from build123d import *

# Parameters (mm, degrees)
F0_R           = 6.35
F1_DEPTH       = 5
F3_D           = 8
F3_CSINK_D     = 10
F3_CSINK_ANGLE = 90


with BuildPart() as f1:
    # F0 (on Top) → F1 (new body)
    with BuildSketch(Plane.XY):
        with BuildLine():
            Line((-10, 65), (-10, 23.348662))
            ThreePointArc((-10, 23.348662), (-21.997045, 12.7), (-25.220534, -3.014077))
            Line((-25.220534, -3.014077), (-61.291651, -23.839746))
            Line((-61.291651, -23.839746), (-51.291651, -41.160254))
            Line((-51.291651, -41.160254), (-15.220534, -20.334585))
            ThreePointArc((-15.220534, -20.334585), (0, -25.4), (15.220534, -20.334585))
            Line((15.220534, -20.334585), (51.291651, -41.160254))
            Line((51.291651, -41.160254), (61.291651, -23.839746))
            Line((61.291651, -23.839746), (25.220534, -3.014077))
            ThreePointArc((25.220534, -3.014077), (21.997045, 12.7), (10, 23.348662))
            Line((10, 23.348662), (10, 65))
            Line((10, 65), (-10, 65))
        make_face()
        with Locations((-12.990381, -7.5)):
            Circle(F0_R, mode=Mode.SUBTRACT)
        with Locations((12.990381, -7.5)):
            Circle(F0_R, mode=Mode.SUBTRACT)
        with Locations((0, 15)):
            Circle(F0_R, mode=Mode.SUBTRACT)
    extrude(amount=F1_DEPTH)

    # F3 (through all)
    with Locations(Plane.XY.offset(5)):
        with Locations((0, 57), (0, 41), (35.507042, -20.5), (49.363448, -28.5), (-35.507042, -20.5), (-49.363448, -28.5)):
            CounterSinkHole(F3_D / 2, F3_CSINK_D / 2, counter_sink_angle=F3_CSINK_ANGLE)


solid = f1.part
Geometry: final body of the model. Coordinates: model frame, mm. A direction names the side the tool comes from. Give positions to 0.01 mm unless a question says otherwise; leave off trailing zeros. Loops run counter-clockwise (first coordinate to the right, second up) from the corner with the lowest first, then second, coordinate; pieces in that order, holes last. Notation, with made-up numbers: M 79.5,-8 L 127.5,-8 A15 ccw 127.5,19 Z; hole C 36.5,8 d8. An arc over 180 degrees is marked long. Put each result on its own line as item: value. Start each with the question number.
1) Ray query, line 1 along Y through (x, z) = (0, 2.7); line 2 along X through (y, z) = (-7, 2); line 3 along X through (y, z) = (-20.5, 3.1). Return the intervals inside material, ascending.
2) Access query for faces 1 (the flat face through (10, 44, 2)), 2 (the flat face through (-10, 44, 2)), 3 (the flat face through (-33.509, -30.893, 2.465)), 4 (the cylindrical face through (0.867, 53.095, 1.972)). Directions: +Z, -Z, +X, -X, +Y, -Y. A direction counts if a zero-diameter tool reaches every point of the face in a straight line with its end or side. Return the directions, or none.
3) Contact query for flat-ended pins moving along their axis: pin 1 (6.5 mm diameter, centred on x = 49.36, y = -28.5, fed in from -Z); pin 2 (2 mm diameter, centred on x = 47.5, z = 4.5, fed in from +Y); pin 3 (3 mm diameter, centred on x = -33.5, z = 3.5, fed in from +Y); pin 4 (3 mm diameter, centred on x = -45, z = 2.5, fed in from +Y). Output: stop coordinate, or through.
4) Cut plane B-B (y = 41). Output: boundary loops of the cut face in (x, z), then the cut area to 3 significant figures.
5) Cut plane D-D (y = 15). Output: boundary loops of the cut face in (x, z), then the cut area to 3 significant figures.
6) Pull-direction query (Y, two-part tool) for faces 5 (the cylindrical face through (53.36, -28.32, 1.97)), 6 (the flat face through (56.222, -32.621, 2.465)), 7 (the flat face through (0, 4, 0)); classes: pulls with the +Y half, pulls with the -Y half, needs draft (parallel to the pull), parting line crosses it, or undercut.
7) Cut plane C-C (y = -7.5). Output: boundary loops of the cut face in (x, z), then the cut area to 3 significant figures.
8) Cut plane A-A (z = 3.25). Give the number of separate pieces and of enclosed holes in the cut face, then the cut area to 3 significant figures.
Verdict:
1. line 1: -25.4 to 8.65, 21.35 to 37, 45 to 53, 61 to 65
1. line 2: -32.12 to -19.32, -6.66 to 6.66, 19.32 to 32.12
1. line 3: -55.51 to -39.51, -31.51 to -15.51, -15 to 15, 15.51 to 31.51, 39.51 to 55.51
2. face 1: +Z, -Z, +X, +Y
2. face 2: +Z, -Z, -X, +Y
2. face 3: +Z, -Z, -Y
2. face 4: +Z, -Z
3. pin 1: through
3. pin 2: y = -15.3
3. pin 3: y = -6.93
3. pin 4: y = -13.57
4. outline: M -10,0 L -4,0 L -4,4 L -5,5 L -10,5 Z; M 4,0 L 10,0 L 10,5 L 5,5 L 4,4 Z
4. area: 59.0 mm2
5. outline: M -20.5,0 L -6.35,0 L -6.35,5 L -20.5,5 Z; M 6.35,0 L 20.5,0 L 20.5,5 L 6.35,5 Z
5. area: 141 mm2
6. face 5: undercut
6. face 6: pulls with the -Y half
6. face 7: needs draft
7. outline: M -32.99,0 L -19.34,0 L -19.34,5 L -32.99,5 Z; M -6.64,0 L 6.64,0 L 6.64,5 L -6.64,5 Z; M 19.34,0 L 32.99,0 L 32.99,5 L 19.34,5 Z
7. area: 203 mm2
8. separate pieces: 1
8. enclosed holes: 9
8. area: 3,760 mm2
